The model under review builds one solid part; all positions refer to its coordinate system, in mm. Face numbers are marked on the shaded views. A direction names the side the tool comes from. Coordinates: 2 decimals unless noted, no trailing zeros. Write each loop counter-clockwise with the first axis right and the second up, starting at its lowest first coordinate (ties: lowest second). Pieces come first, ordered by that corner, then holes.
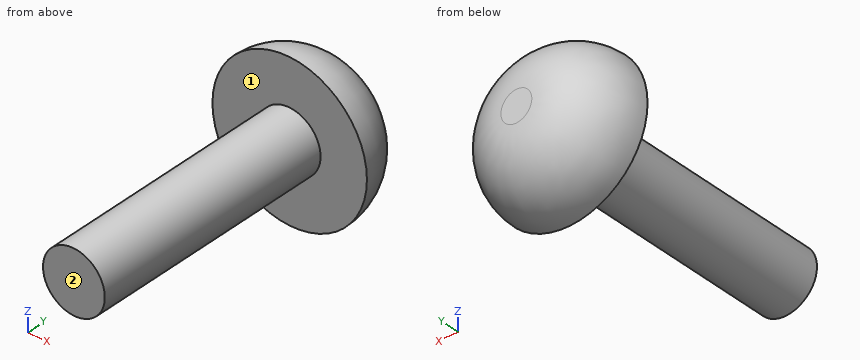
Autodesk Inventor part; units mm, degrees
ref_plane "YZ Plane" through (0, 0, 0) normal (1, 0, 0) x (0, 1, 0)
ref_plane "XZ Plane" through (0, 0, 0) normal (0, 1, 0) x (-1, 0, 0)
ref_plane "XY Plane" through (0, 0, 0) normal (0, 0, 1) x (1, 0, 0)
sketch "Sketch1" plane through (0, 0, 0) normal (0, 1, 0) x (-1, 0, 0)
  circle A0 centre (0, 0) radius 0.7937
  dimension "d0" = 1.5875
extrude "Extrusion1" add sketch "Sketch1" along normal blind 6.35
sketch "Sketch2" plane through (0, 6.35, 0) normal (0, 1, 0) x (1, 0, 0)
  circle A0 centre (0, 0) radius 0.7937
  circle A1 centre (0, 0) radius 1.9837
  dimension "d3" = 3.9675
extrude "Extrusion2" add sketch "Sketch2" along normal blind 1.5875
sketch "Sketch3" plane through (0, 6.35, 0) normal (0, 1, 0) x (1, 0, 0)
  circle A0 centre (0, 0) radius 0.7937
extrude "Extrusion3" add sketch "Sketch3" along normal blind 1.5875
fillet "Fillet1" radius 1.5875 1 edges at (-1.9837, 7.9375, 0)
properties part number "linkage peg"
Item 1: To check wall thickness, follow line 1 along X through (y, z) = (7.5, -0.5); line 2 along Y through (x, z) = (-0.6, 1.75); line 3 along X through (y, z) = (5.5, -0.35). State the ranges of each line that lie inside material, in increasing order.
Solved:
line 1: x = -1.4 to 1.4
line 2: y = 6.35 to 6.99
line 3: x = -0.71 to 0.71
Item 2: For pin 1 (1 mm diameter, centred on y = 3.5, z = -1, fed in from -X); pin 2 (1 mm diameter, centred on y = 7, z = -0.5, fed in from -X), all flat-tipped, find the tip position at first contact; note any pin that passes through.
Solved:
pin 1: stops at x = -0.62
pin 2: stops at x = -1.95
Item 3: Take a section at A-A, the plane y = 5. Write out the cut boundary in (x, z), plus the area to 3 significant figures.
Solved:
outline: circle Ø1.59 at (0, 0)
area: 1.98 mm2
Item 4: Machinability: for the marked faces 1 and 2, which of the approach directions +Z, -Z, +X, -X, +Y, -Y give a long, thin tool a straight path to every point of the face, cutting with its end or side? Answer none if there is none.
Solved:
face 1: -Y
face 2: +Z, -Z, +X, -X, -Y
